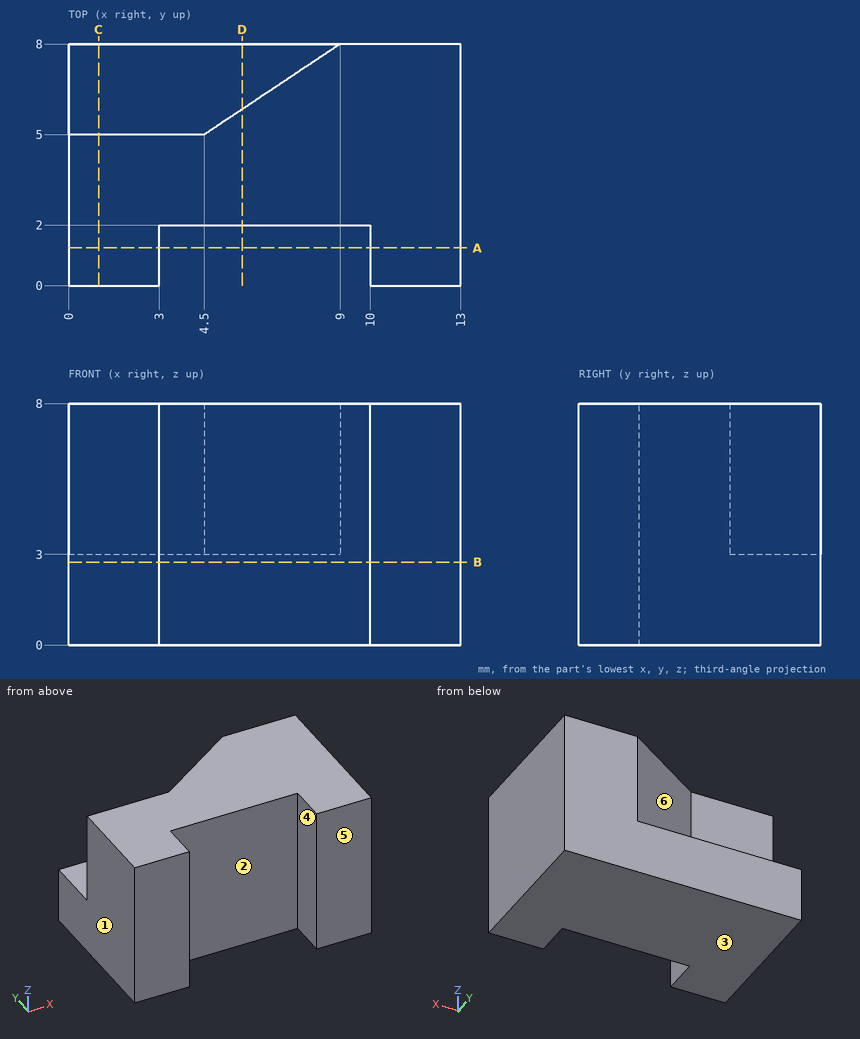
Geometry check sheet. Reference: drawing and pictorial views, mm from the part's lowest x, y, z. A direction names the side the tool comes from. Round coordinates to 2 decimals unless told otherwise and drop trailing zeros. Order: outer loops, then holes, each group sorted by start corner. A loop starts at its lowest first (then second) coordinate and runs counter-clockwise, first axis right, second up. Notation, with made-up numbers: M 83,65 L 116,65 A3 cw 116,70 Z; hole C 27,23.5 d7. An arc over 180 degrees is marked long. Answer in a Markdown table with one row per item.
(1) Sectioned sample at C-C, the plane x = 1. Record the cut outline in (y, z), and give its area (3 significant figures).
Responses:
| item | result |
|---|---|
| outline | M 0,0 L 8,0 L 8,3 L 5,3 L 5,8 L 0,8 Z |
| area | 49.0 mm² |
(2) Scan lines: probe 1 along X at (y, z) = (1.5, 5.5); probe 2 along Z at (x, y) = (5.25, 7.5); probe 3 along Y at (x, z) = (6, 0.75). Record each from-to range of solid material in increasing order. Write a range as from..to.
Responses:
| item | result |
|---|---|
| probe 1 | x = 0..3, 10..13 |
| probe 2 | z = 0..3 |
| probe 3 | y = 2..8 |
(3) Draft check along X on the marked faces 1, 2, 3 and 4. Enter one of: released by +X, released by -X, zero draft, split by the parting line, or undercut.
Responses:
| item | result |
|---|---|
| face 1 | released by -X |
| face 2 | undercut |
| face 3 | zero draft |
| face 4 | undercut |
(4) Tool access check on the marked faces 5 and 6. Record the directions out of +Z, -Z, +X, -X, +Y, -Y that give a thin tool (end or side, any length) a straight path to the whole face; none if there is none.
Responses:
| item | result |
|---|---|
| face 5 | +Z, -Z, +X, -X, -Y |
| face 6 | +Z, -X, +Y |
(5) Sectioned sample at D-D, the plane x = 5.75. Record the cut outline in (y, z), and give its area (3 significant figures).
Responses:
| item | result |
|---|---|
| outline | M 2,0 L 8,0 L 8,3 L 5.83,3 L 5.83,8 L 2,8 Z |
| area | 37.2 mm² |
(6) Sectioned sample at A-A, the plane y = 1.25. Record the cut outline in (x, z).
Responses:
| item | result |
|---|---|
| outline | M 0,0 L 3,0 L 3,8 L 0,8 Z; M 10,0 L 13,0 L 13,8 L 10,8 Z |
(7) Sectioned sample at B-B, the plane z = 2.75. Record the cut outline in (x, y), and give its area (3 significant figures).
Responses:
| item | result |
|---|---|
| outline | M 0,0 L 3,0 L 3,2 L 10,2 L 10,0 L 13,0 L 13,8 L 0,8 Z |
| area | 90.0 mm² |
(8) Go/stop test with a flat-tipped pin: P1, Ø0.9, axis at x = 3.5, y = 7, coming from the +Z side. Record where the tip stops, or that it passes through.
Responses:
| item | result |
|---|---|
| P1 | stops at z = 3 |
